Read the model definition and answer for the solid it produces. Units are mm, in the model's axes. Coordinates: 2 decimals unless noted, no trailing zeros. Loops run counter-clockwise (first coordinate to the right, second up) from the corner with the lowest first, then second, coordinate; pieces in that order, holes last. Notation, with made-up numbers: (-12, 78) -> (-2, 78) arc R17 ccw to (-2, 99) -> close; hole circle Ø2 at (-18, -11). An arc over 180 degrees is marked (long way). Answer as a JSON object with one key per item and string values. Group by question number.
1) Section A-A, the plane x = 0 is taken. Give the vertices of the cut face in (y, z).
2) Flat-ended cylindrical pins translate along their axes: P1, Ø3, axis at x = 51.5, y = 64.5, coming from the +Z side; P2, Ø3.5, axis at x = -5, z = -64, coming from the +Y side; P3, Ø1.5, axis at y = 73.5, z = -22.5, coming from the +X side. Find the tip coordinate at first contact, or state that the pin passes through.
3) Section C-C, the plane y = 48.5 is taken. Give the vertices of the cut face in (x, z).
4) Section B-B, the plane z = 0 is taken. Give the vertices of the cut face in (x, y).
5) Section D-D, the plane z = -36 is taken. Give the vertices of the cut face in (x, y).
6) Consider probe 1 along X at (y, z) = (27.5, 1); probe 2 along Z at (x, y) = (30.5, 5.5); probe 3 along Z at (x, y) = (-49, 25.5). Determine where each line is inside the solid, lowest interval first. Write a range as [from, to].
from build123d import *

# Parameters (mm, degrees)
SKETCH1_R           = 60
BOSS_EXTRUDE1_DEPTH = 100
BOSS_EXTRUDE2_START = -25
BOSS_EXTRUDE2_DEPTH = 5


with BuildPart() as part:
    # Sketch1 → Boss-Extrude1 (new body)
    with BuildSketch(Plane(origin=(0, 0, 0), x_dir=(1, 0, 0), z_dir=(0, 1, 0))):
        with Locations(Location((0, 0, 0), (0, 0, 270))):
            Circle(SKETCH1_R)
    extrude(amount=BOSS_EXTRUDE1_DEPTH)

    # Sketch2 → Boss-Extrude2 (add)
    with BuildSketch(Plane(origin=(0, 100, 0), x_dir=(1, 0, 0), z_dir=(0, 1, 0)).offset(BOSS_EXTRUDE2_START)):
        with BuildLine():
            ThreePointArc((-10.714427791, 59.035591274), (-42.426406871, 42.426406871), (-59.035591274, 10.714427791))
            ThreePointArc((-59.035591274, 10.714427791), (-61.233489712, 6.767544156), (-65.384615385, 4.985185153))
            ThreePointArc((-65.384615385, 4.985185153), (-70, 0), (-65.384615385, -4.985185153))
            ThreePointArc((-65.384615385, -4.985185153), (-61.233489712, -6.767544156), (-59.035591274, -10.714427791))
            ThreePointArc((-59.035591274, -10.714427791), (-42.426406871, -42.426406871), (-10.714427791, -59.035591274))
            ThreePointArc((-10.714427791, -59.035591274), (-6.767544156, -61.233489712), (-4.985185153, -65.384615385))
            ThreePointArc((-4.985185153, -65.384615385), (0, -70), (4.985185153, -65.384615385))
            ThreePointArc((4.985185153, -65.384615385), (6.767544156, -61.233489712), (10.714427791, -59.035591274))
            ThreePointArc((10.714427791, -59.035591274), (42.426406871, -42.426406871), (59.035591274, -10.714427791))
            ThreePointArc((59.035591274, -10.714427791), (61.233489712, -6.767544156), (65.384615385, -4.985185153))
            ThreePointArc((65.384615385, -4.985185153), (70, 0), (65.384615385, 4.985185153))
            ThreePointArc((65.384615385, 4.985185153), (61.233489712, 6.767544156), (59.035591274, 10.714427791))
            ThreePointArc((59.035591274, 10.714427791), (42.426406871, 42.426406871), (10.714427791, 59.035591274))
            ThreePointArc((10.714427791, 59.035591274), (6.767544156, 61.233489712), (4.985185153, 65.384615385))
            ThreePointArc((4.985185153, 65.384615385), (0, 70), (-4.985185153, 65.384615385))
            ThreePointArc((-4.985185153, 65.384615385), (-6.767544156, 61.233489712), (-10.714427791, 59.035591274))
        make_face()
    extrude(amount=BOSS_EXTRUDE2_DEPTH)


solid = part.part
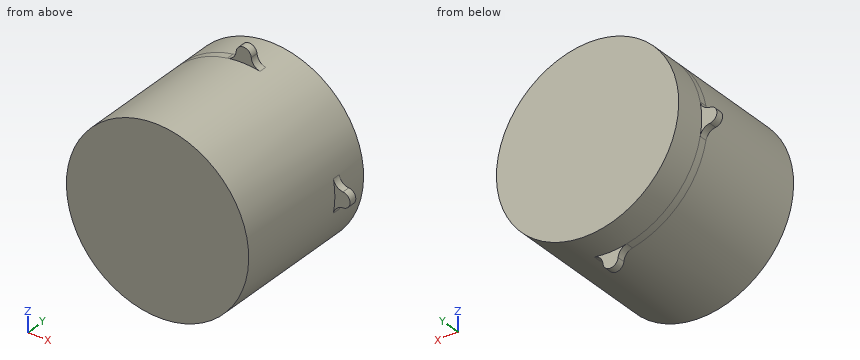
Determined:
{
 "1": {"outline": "(0, -60) -> (75, -60) -> (75, -70) -> (80, -70) -> (80, -60) -> (100, -60) -> (100, 60) -> (80, 60) -> (80, 70) -> (75, 70) -> (75, 60) -> (0, 60) -> close"},
 "2": {"P1": "z = 33.17", "P2": "y = 80", "P3": "x = 55.92"},
 "3": {"outline": "circle Ø120 at (0, 0)"},
 "4": {"outline": "(-70, 75) -> (-60, 75) -> (-60, 0) -> (60, 0) -> (60, 75) -> (70, 75) -> (70, 80) -> (60, 80) -> (60, 100) -> (-60, 100) -> (-60, 80) -> (-70, 80) -> close"},
 "5": {"outline": "(-48, 0) -> (48, 0) -> (48, 100) -> (-48, 100) -> close"},
 "6": {"probe 1": "[-59.99, 59.99]", "probe 2": "[-51.67, 51.67]", "probe 3": "[-34.63, 34.63]"}
}
